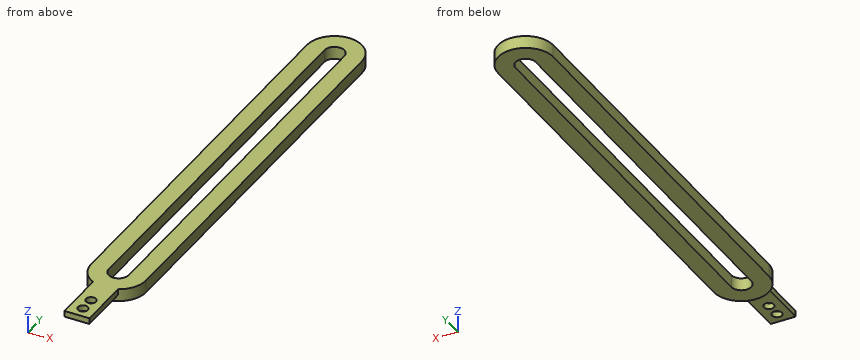
```python
from build123d import *

# Parameters (mm, degrees)
BOSS_EXTRUDE1_DEPTH = 5
BOSS_EXTRUDE2_START = -2.4
BOSS_EXTRUDE2_DEPTH = 2.4
SKETCH3_R           = 2
CUT_EXTRUDE1_DEPTH  = 2.4


with BuildPart() as part:
    # Sketch1 → Boss-Extrude1 (new body)
    with BuildSketch(Plane.XY):
        with BuildLine():
            Line((11, 0), (11, -160))
            ThreePointArc((11, -160), (0, -171), (-11, -160))
            Line((-11, -160), (-11, 0))
            ThreePointArc((-11, 0), (0, 11), (11, 0))
        make_face()
        with BuildLine():
            Line((-4, -160), (-4, 0))
            ThreePointArc((-4, 0), (0, 4), (4, 0))
            Line((4, 0), (4, -160))
            ThreePointArc((4, -160), (0, -164), (-4, -160))
        make_face(mode=Mode.SUBTRACT)
    extrude(amount=BOSS_EXTRUDE1_DEPTH)

    # Sketch2 → Boss-Extrude2 (add)
    with BuildSketch(Plane.XY.offset(5).offset(BOSS_EXTRUDE2_START)):
        with BuildLine():
            Line((-5, -171), (-5, -169.797958971))
            ThreePointArc((-5, -169.797958971), (0, -171), (5, -169.797958971))
            Line((5, -169.797958971), (5, -171))
            Line((5, -171), (5, -191))
            Line((5, -191), (-5, -191))
            Line((-5, -191), (-5, -171))
        make_face()
    extrude(amount=BOSS_EXTRUDE2_DEPTH)

    # Sketch3 → Cut-Extrude1 (cut)
    with BuildSketch(Plane(origin=(0, 0, 2.6), x_dir=(-1, 0, 0), z_dir=(0, 0, -1))):
        with Locations((0, -186.5)):
            Circle(SKETCH3_R)
        with Locations((0, -180.5)):
            Circle(SKETCH3_R)
    extrude(amount=-CUT_EXTRUDE1_DEPTH, mode=Mode.SUBTRACT)


solid = part.part
```
The listing builds one solid part. Answer for the finished solid, in the listing's coordinates (mm). Give positions to 0.01 mm unless a question says otherwise; leave off trailing zeros. Order: outer loops, then holes, each group sorted by start corner. A loop starts at its lowest first (then second) coordinate and runs counter-clockwise, first axis right, second up. Notation, with made-up numbers: M 77.25,51.25 L 119.25,51.25 A30 cw 119.25,82.25 Z; hole C 27.5,-7 d10. An arc over 180 degrees is marked long. Put each result on its own line as item: value. Start each with the question number.
Item 1: The part is cut by section B-B, the plane y = -114. Determine the outline of the cut face in (x, z), and give its area (3 significant figures).
Item 2: Flat-ended cylindrical pins translate along their axes: P1, Ø3, axis at x = 0, y = -180.5, coming from the -Z side; P2, Ø5, axis at x = 0, y = -186.5, coming from the -Z side; P3, Ø1.9, axis at y = -179, z = 4, coming from the -X side; P4, Ø10, axis at x = -2.5, y = -42.5, coming from the +Z side. Find the tip coordinate at first contact, or state that the pin passes through.
Item 3: The part is cut by section A-A, the plane x = 0. Determine the outline of the cut face in (y, z).
Item 4: Find the intervals of material crossed by line 1 along Y through (x, z) = (0, 3.35); line 2 along X through (y, z) = (-186.5, 4.4); line 3 along X through (y, z) = (-104.5, 1.45), in increasing order.
Item 5: The part is cut by section D-D, the plane y = -186.5. Determine the outline of the cut face in (x, z).
Item 6: The part is cut by section C-C, the plane z = 1.65. Determine the outline of the cut face in (x, y).
Answer key:
1. outline: M -11,0 L -4,0 L -4,5 L -11,5 Z; M 4,0 L 11,0 L 11,5 L 4,5 Z
1. area: 70.0 mm²
2. P1: passes through
2. P2: stops at z = 2.6
2. P3: stops at x = -5
2. P4: stops at z = 5
3. outline: M -191,2.6 L -188.5,2.6 L -188.5,5 L -191,5 Z; M -184.5,2.6 L -182.5,2.6 L -182.5,5 L -184.5,5 Z; M -178.5,2.6 L -171,2.6 L -171,0 L -164,0 L -164,5 L -178.5,5 Z; M 4,0 L 11,0 L 11,5 L 4,5 Z
4. line 1: y = -191 to -188.5, -184.5 to -182.5, -178.5 to -164, 4 to 11
4. line 2: x = -5 to -2, 2 to 5
4. line 3: x = -11 to -4, 4 to 11
5. outline: M -5,2.6 L -2,2.6 L -2,5 L -5,5 Z; M 2,2.6 L 5,2.6 L 5,5 L 2,5 Z
6. outline: M -11,-160 A11 ccw 11,-160 L 11,0 A11 ccw -11,0 Z; hole M -4,-160 A4 ccw 4,-160 L 4,0 A4 ccw -4,0 Z
